from build123d import *

# Parameters (mm, degrees)
SKETCH2_W           = 28.575
SKETCH2_H           = 292.1
BOSS_EXTRUDE1_DEPTH = 6.35
SKETCH4_R           = 6.35
CUT_EXTRUDE1_DEPTH  = 7.35
SKETCH5_R           = 7.9375
CUT_EXTRUDE2_DEPTH  = 1.5875


with BuildPart() as part:
    # Sketch2 → Boss-Extrude1 (new body, symmetric)
    with BuildSketch(Plane.XY):
        with Locations((0, 127)):
            Rectangle(SKETCH2_W, SKETCH2_H)
    extrude(amount=BOSS_EXTRUDE1_DEPTH, both=True)

    # Sketch4 → Cut-Extrude1 (cut, symmetric)
    with BuildSketch(Plane.XY):
        Circle(SKETCH4_R)
    cut_extrude1 = extrude(amount=CUT_EXTRUDE1_DEPTH, both=True, mode=Mode.SUBTRACT)

    # Sketch5 → Cut-Extrude2 (cut)
    with BuildSketch(Plane.XY.offset(6.35)):
        Circle(SKETCH5_R)
    cut_extrude2 = extrude(amount=-CUT_EXTRUDE2_DEPTH, mode=Mode.SUBTRACT)

    # Mirror1: Cut-Extrude1, Cut-Extrude2 across plane
    add(cut_extrude1.mirror(Plane(origin=(0, 127, 0), x_dir=(0, 0, 1), z_dir=(0, -1, 0))), mode=Mode.SUBTRACT)
    add(cut_extrude2.mirror(Plane(origin=(0, 127, 0), x_dir=(0, 0, 1), z_dir=(0, -1, 0))), mode=Mode.SUBTRACT)


solid = part.part
Geometry check sheet. Reference: the model listing, model coordinates, mm. A direction names the side the tool comes from. Give positions to 0.01 mm unless a question says otherwise; leave off trailing zeros. Order: outer loops, then holes, each group sorted by start corner. A loop starts at its lowest first (then second) coordinate and runs counter-clockwise, first axis right, second up. Notation, with made-up numbers: M 57,52.25 L 66,52.25 A32 ccw 66,83.25 Z; hole C -2.5,-35.75 d7. An arc over 180 degrees is marked long. Use a Markdown table: item, result.
Item 1: Section check A-A (y = 0). Record the cut outline in (x, z), and give its area (3 significant figures).
Answers follow:
| item | result |
|---|---|
| outline | M -14.29,-6.35 L -6.35,-6.35 L -6.35,4.76 L -7.94,4.76 L -7.94,6.35 L -14.29,6.35 Z; M 6.35,-6.35 L 14.29,-6.35 L 14.29,6.35 L 7.94,6.35 L 7.94,4.76 L 6.35,4.76 Z |
| area | 197 mm2 |
Item 2: Material ranges on line 1 along Y through (x, z) = (0, 6); line 2 along Y through (x, z) = (0, -4); line 3 along X through (y, z) = (254, 5.4), recorded low to high.
Answers follow:
| item | result |
|---|---|
| line 1 | y = -19.05 to -7.94, 7.94 to 246.06, 261.94 to 273.05 |
| line 2 | y = -19.05 to -6.35, 6.35 to 247.65, 260.35 to 273.05 |
| line 3 | x = -14.29 to -7.94, 7.94 to 14.29 |
Item 3: Section check B-B (z = 2). Record the cut outline in (x, y), and give its area (3 significant figures).
Answers follow:
| item | result |
|---|---|
| outline | M -14.29,-19.05 L 14.29,-19.05 L 14.29,273.05 L -14.29,273.05 Z; hole C 0,0 d12.7; hole C 0,254 d12.7 |
| area | 8,090 mm2 |
Item 4: Draft check along X on faces 3 (the flat face through (14.288, 125, 0)), 4 (the flat face through (0, 7, 4.762)), 5 (the flat face through (0, 129, 6.35)), 6 (the cylindrical face through (-6.3, 258.83, 5.57)). Enter one of: +X half, -X half, draft (parallel to the pull), parting line (faces both ways), or undercut.
Answers follow:
| item | result |
|---|---|
| face 3 | +X half |
| face 4 | undercut |
| face 5 | draft |
| face 6 | undercut |
Item 5: Tool access check on faces 1 (the cylindrical face through (-1.38, -6.2, -0.72)), 2 (the cylindrical face through (-1.72, -7.75, 5.57)). Record the directions out of +Z, -Z, +X, -X, +Y, -Y that give a thin tool (end or side, any length) a straight path to the whole face; none if there is none.
Answers follow:
| item | result |
|---|---|
| face 1 | +Z, -Z |
| face 2 | +Z |
Item 6: Section check C-C (x = 0). Record the cut outline in (y, z), and give its area (3 significant figures).
Answers follow:
| item | result |
|---|---|
| outline | M -19.05,-6.35 L -6.35,-6.35 L -6.35,4.76 L -7.94,4.76 L -7.94,6.35 L -19.05,6.35 Z; M 6.35,-6.35 L 247.65,-6.35 L 247.65,4.76 L 246.06,4.76 L 246.06,6.35 L 7.94,6.35 L 7.94,4.76 L 6.35,4.76 Z; M 260.35,-6.35 L 273.05,-6.35 L 273.05,6.35 L 261.94,6.35 L 261.94,4.76 L 260.35,4.76 Z |
| area | 3,380 mm2 |
